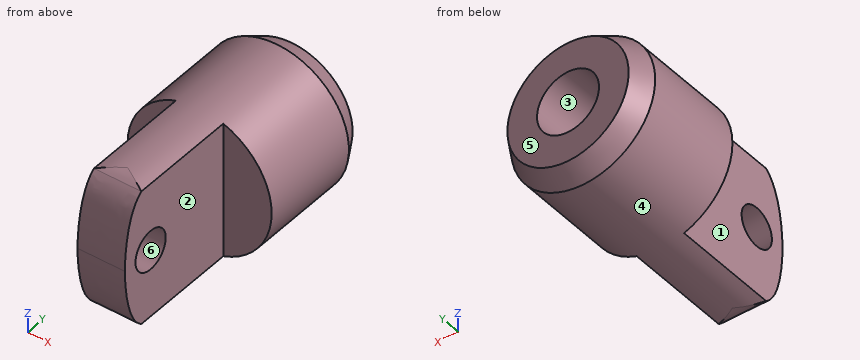
from build123d import *

# Parameters (mm, degrees)
SKETCH3_R                           = 4.6355
BOSS_EXTRUDE1_DEPTH                 = 8.001
SKETCH4_R                           = 1.9939
CUT_EXTRUDE1_DEPTH                  = 5.588
CHAMFER1_SIZE                       = 1.27
CHAMFER1_SIZE2                      = 0.733234842
CUT_EXTRUDE2_REACH                  = 12.344
CUT_EXTRUDE2_END_RADIUS             = 4.6355
SKETCH5_W                           = 3.887671843
SKETCH5_H                           = 8.255
CUT_EXTRUDE2_DIRECTION_2_REACH      = 12.344
CUT_EXTRUDE2_DIRECTION_2_END_RADIUS = 4.6355
CUT_EXTRUDE3_REACH                  = 13.111
CUT_EXTRUDE4_REACH                  = 13.111
SKETCH7_R                           = 1.27


with BuildPart() as part:
    # Sketch3 → Boss-Extrude1 (new, symmetric)
    with BuildSketch(Plane(origin=(0, 0, 0), x_dir=(1, 0, 0), z_dir=(0, 1, 0))):
        with Locations(Location((0, 0, 0), (0, 0, 270))):
            Circle(SKETCH3_R)
    extrude(amount=BOSS_EXTRUDE1_DEPTH, both=True)

    # Sketch4 → Cut-Extrude1 (cut)
    with BuildSketch(Plane(origin=(0, 8.001, 0), x_dir=(1, 0, 0), z_dir=(0, 1, 0))):
        with Locations(Location((0, 0, 0), (0, 0, 270))):
            Circle(SKETCH4_R)
    extrude(amount=-CUT_EXTRUDE1_DEPTH, mode=Mode.SUBTRACT)

    # Chamfer1
    chamfer1_edges = [part.edges().sort_by_distance(p)[0] for p in [
        (0, 8.001, -4.6355),
    ]]
    chamfer1_side = [part.faces().sort_by_distance(p)[0] for p in [
        (0, 0, -4.6355),
    ]]
    chamfer(chamfer1_edges, length=CHAMFER1_SIZE, length2=CHAMFER1_SIZE2, reference=chamfer1_side[0])

    # Cut-Extrude2: up to this cylinder (the profile starts inside it)
    cut_extrude2_end = Plane(origin=(0, -3.8735, 0), z_dir=(0, -1, 0)) * Cylinder(CUT_EXTRUDE2_END_RADIUS, 34.959, mode=Mode.PRIVATE)
    # Sketch5 → Cut-Extrude2 (cut, up to the surface)
    with BuildSketch(Plane.XY, mode=Mode.PRIVATE) as cut_extrude2_sk1:
        with Locations((-3.467835922, -3.8735)):
            Rectangle(SKETCH5_W, SKETCH5_H)
    cut_extrude2_tool1 = extrude(cut_extrude2_sk1.sketch, amount=-CUT_EXTRUDE2_REACH, mode=Mode.PRIVATE) & cut_extrude2_end
    add(cut_extrude2_tool1.solids().sort_by_distance((-3.467836, -3.8735, 0))[0], mode=Mode.SUBTRACT)
    # Sketch5 → Cut-Extrude2 (cut, up to the surface)
    with BuildSketch(Plane.XY, mode=Mode.PRIVATE) as cut_extrude2_sk2:
        with Locations((3.467835922, -3.8735)):
            Rectangle(SKETCH5_W, SKETCH5_H)
    cut_extrude2_tool2 = extrude(cut_extrude2_sk2.sketch, amount=-CUT_EXTRUDE2_REACH, mode=Mode.PRIVATE) & cut_extrude2_end
    add(cut_extrude2_tool2.solids().sort_by_distance((3.467836, -3.8735, 0))[0], mode=Mode.SUBTRACT)

    # Cut-Extrude2 direction 2: up to this cylinder (the profile starts inside it)
    cut_extrude2_direction_2_end = Plane(origin=(0, -3.8735, 0), z_dir=(0, -1, 0)) * Cylinder(CUT_EXTRUDE2_DIRECTION_2_END_RADIUS, 34.959, mode=Mode.PRIVATE)
    # Sketch5 → Cut-Extrude2 direction 2 (cut, up to the surface)
    with BuildSketch(Plane.XY, mode=Mode.PRIVATE) as cut_extrude2_direction_2_sk1:
        with Locations((-3.467835922, -3.8735)):
            Rectangle(SKETCH5_W, SKETCH5_H)
    cut_extrude2_direction_2_tool1 = extrude(cut_extrude2_direction_2_sk1.sketch, amount=CUT_EXTRUDE2_DIRECTION_2_REACH, mode=Mode.PRIVATE) & cut_extrude2_direction_2_end
    add(cut_extrude2_direction_2_tool1.solids().sort_by_distance((-3.467836, -3.8735, 0))[0], mode=Mode.SUBTRACT)
    # Sketch5 → Cut-Extrude2 direction 2 (cut, up to the surface)
    with BuildSketch(Plane.XY, mode=Mode.PRIVATE) as cut_extrude2_direction_2_sk2:
        with Locations((3.467835922, -3.8735)):
            Rectangle(SKETCH5_W, SKETCH5_H)
    cut_extrude2_direction_2_tool2 = extrude(cut_extrude2_direction_2_sk2.sketch, amount=CUT_EXTRUDE2_DIRECTION_2_REACH, mode=Mode.PRIVATE) & cut_extrude2_direction_2_end
    add(cut_extrude2_direction_2_tool2.solids().sort_by_distance((3.467836, -3.8735, 0))[0], mode=Mode.SUBTRACT)

    # Sketch6 → Cut-Extrude3 (cut, up to next)
    with BuildSketch(Plane(origin=(1.524, 0, 0), x_dir=(0, 0, -1), z_dir=(1, 0, 0)), mode=Mode.PRIVATE) as cut_extrude3_sk1:
        with BuildLine():
            add(Edge.make_bspline(
                [(-4.377817293, -6.618376883), (-3.503121267, -7.894799124), (-0.664999949, -8.001), (0, -8.001)],
                knots=[0.156984914, 0.156984914, 0.156984914, 0.156984914, 1, 1, 1, 1], degree=3))
            Line((-4.377817293, -6.618376883), (-4.377817293, -8.001))
            Line((-4.377817293, -8.001), (0, -8.001))
        make_face()
    cut_extrude3_tool1 = extrude(cut_extrude3_sk1.sketch, amount=-CUT_EXTRUDE3_REACH, mode=Mode.PRIVATE) & part.part
    # Sketch6 → Cut-Extrude3 (cut, up to next)
    with BuildSketch(Plane(origin=(1.524, 0, 0), x_dir=(0, 0, -1), z_dir=(1, 0, 0)), mode=Mode.PRIVATE) as cut_extrude3_sk2:
        with BuildLine():
            add(Edge.make_bspline(
                [(4.377817293, -6.618376883), (3.503121267, -7.894799124), (0.664999949, -8.001), (0, -8.001)],
                knots=[0.156984914, 0.156984914, 0.156984914, 0.156984914, 1, 1, 1, 1], degree=3))
            Line((0, -8.001), (4.377817293, -8.001))
            Line((4.377817293, -8.001), (4.377817293, -6.618376883))
        make_face()
    cut_extrude3_tool2 = extrude(cut_extrude3_sk2.sketch, amount=-CUT_EXTRUDE3_REACH, mode=Mode.PRIVATE) & part.part
    # Sketch6 → Cut-Extrude3 (cut, up to next)
    with BuildSketch(Plane(origin=(1.524, 0, 0), x_dir=(0, 0, -1), z_dir=(1, 0, 0)), mode=Mode.PRIVATE) as cut_extrude3_sk3:
        with BuildLine():
            add(Edge.make_bspline(
                [(-4.6355, -5.776685713), (-4.6355, -6.102410184), (-4.54070178, -6.380683586), (-4.377817293, -6.618376883)],
                knots=[0, 0, 0, 0, 0.156984914, 0.156984914, 0.156984914, 0.156984914], degree=3))
            Line((-4.6355, -5.776685713), (-4.6355, -8.001))
            Line((-4.6355, -8.001), (-4.377817293, -8.001))
            Line((-4.377817293, -8.001), (-4.377817293, -6.618376883))
        make_face()
    cut_extrude3_tool3 = extrude(cut_extrude3_sk3.sketch, amount=-CUT_EXTRUDE3_REACH, mode=Mode.PRIVATE) & part.part
    # Sketch6 → Cut-Extrude3 (cut, up to next)
    with BuildSketch(Plane(origin=(1.524, 0, 0), x_dir=(0, 0, -1), z_dir=(1, 0, 0)), mode=Mode.PRIVATE) as cut_extrude3_sk4:
        with BuildLine():
            Line((4.6355, -8.001), (4.6355, -5.776685713))
            add(Edge.make_bspline(
                [(4.6355, -5.776685713), (4.6355, -6.102410184), (4.54070178, -6.380683586), (4.377817293, -6.618376883)],
                knots=[0, 0, 0, 0, 0.156984914, 0.156984914, 0.156984914, 0.156984914], degree=3))
            Line((4.377817293, -6.618376883), (4.377817293, -8.001))
            Line((4.377817293, -8.001), (4.6355, -8.001))
        make_face()
    cut_extrude3_tool4 = extrude(cut_extrude3_sk4.sketch, amount=-CUT_EXTRUDE3_REACH, mode=Mode.PRIVATE) & part.part
    add(cut_extrude3_tool1.solids().sort_by_distance((1.524, -7.641566, 3.372722))[0], mode=Mode.SUBTRACT)
    add(cut_extrude3_tool2.solids().sort_by_distance((1.524, -7.641566, -3.372722))[0], mode=Mode.SUBTRACT)
    add(cut_extrude3_tool3.solids().sort_by_distance((1.524, -7.165384, 4.5152))[0], mode=Mode.SUBTRACT)
    add(cut_extrude3_tool4.solids().sort_by_distance((1.524, -7.165384, -4.5152))[0], mode=Mode.SUBTRACT)

    # Sketch7 → Cut-Extrude4 (cut, up to next)
    with BuildSketch(Plane(origin=(1.524, 0, 0), x_dir=(0, 0, -1), z_dir=(1, 0, 0)), mode=Mode.PRIVATE) as cut_extrude4_sk1:
        with Locations((0, -5.842)):
            Circle(SKETCH7_R)
    cut_extrude4_tool1 = extrude(cut_extrude4_sk1.sketch, amount=-CUT_EXTRUDE4_REACH, mode=Mode.PRIVATE) & part.part
    add(cut_extrude4_tool1.solids().sort_by_distance((1.524, -5.842, 0))[0], mode=Mode.SUBTRACT)


solid = part.part
The listing builds one solid part. Answer for the finished solid, in the listing's coordinates (mm). Face numbers are marked on the shaded views. A direction names the side the tool comes from. Give positions to 0.01 mm unless a question says otherwise; leave off trailing zeros. Loops run counter-clockwise (first coordinate to the right, second up) from the corner with the lowest first, then second, coordinate; pieces in that order, holes last.
Item 1: Determine the mould class of the marked faces 4, 5 and 6 for opening direction Z: +Z half, -Z half, draft (parallel to the pull), parting line (faces both ways), or undercut.
Derived:
face 4: parting line
face 5: draft
face 6: undercut
Item 2: A tool of negligible diameter and unlimited length cuts with its end or side. For the marked faces 1, 2 and 3, from which of +Z, -Z, +X, -X, +Y, -Y can it reach the whole face along a straight path? Write none if from no direction.
Derived:
face 1: +Z, -Z, -X, -Y
face 2: +Z, -Z, +X, -Y
face 3: +Y
Item 3: Each of these flat-tipped pins is pushed along its axis until it touches: pin 1 Ø5 at (x, y) = (-2.5, 1.5) entering from -Z; pin 2 Ø1.6 at (x, z) = (-2.5, -1) entering from -Y; pin 3 Ø1 at (y, z) = (0, 1) entering from -X; pin 4 Ø2.5 at (y, z) = (-4, 0.5) entering from +X. Where does it stop, or does it pass through?
Derived:
pin 1: stops at z = -4.64
pin 2: stops at y = 0.25
pin 3: stops at x = -4.6
pin 4: stops at x = 1.52
Item 4: Find the intervals of material crossed by line 1 along Y through (x, z) = (0.7, 0); line 2 along X through (y, z) = (-2.75, 2); line 3 along Z through (x, y) = (0.75, 5.5), in increasing order.
Derived:
line 1: y = -8 to -7.11, -4.57 to 2.41
line 2: x = -1.52 to 1.52
line 3: z = -4.57 to -1.85, 1.85 to 4.57
Item 5: A cutting plane is placed at A-A (y = -1). Give the vertices of the cut face in (x, z).
Derived:
outline: (-1.52, -4.38) arc R4.64 ccw to (1.52, -4.38) - (1.52, 4.38) arc R4.64 ccw to (-1.52, 4.38) - close
